Source: three-view drawing plus pictorial views. Frame: mm from the lowest corner of the part. Round coordinates to 2 decimals unless told otherwise and drop trailing zeros. Loops run counter-clockwise (first coordinate to the right, second up) from the corner with the lowest first, then second, coordinate; pieces in that order, holes last. Notation, with made-up numbers: (53, 18.25) -> (63, 18.25) arc R12 ccw to (63, 35.25) -> close; hole circle Ø8 at (-28, 29). An arc over 180 degrees is marked (long way). Put each result on its own line as item: value. Start each with the question number.
1. Material intervals for L1, parallel to Z at x = 0.85, y = 1.6; L2, parallel to Z at x = 5.7, y = 2.75; L3, parallel to Y at x = 2.85, z = 12.5, sorted ascending.
2. Cut plane A-A (z = 15). Return the cut outline in (x, y).
3. Contact query for a flat-ended pin moving along its axis: pin 1 (2 mm diameter, centred on y = 1.5, z = 19.5, fed in from +X). Output: stop coordinate, or through.
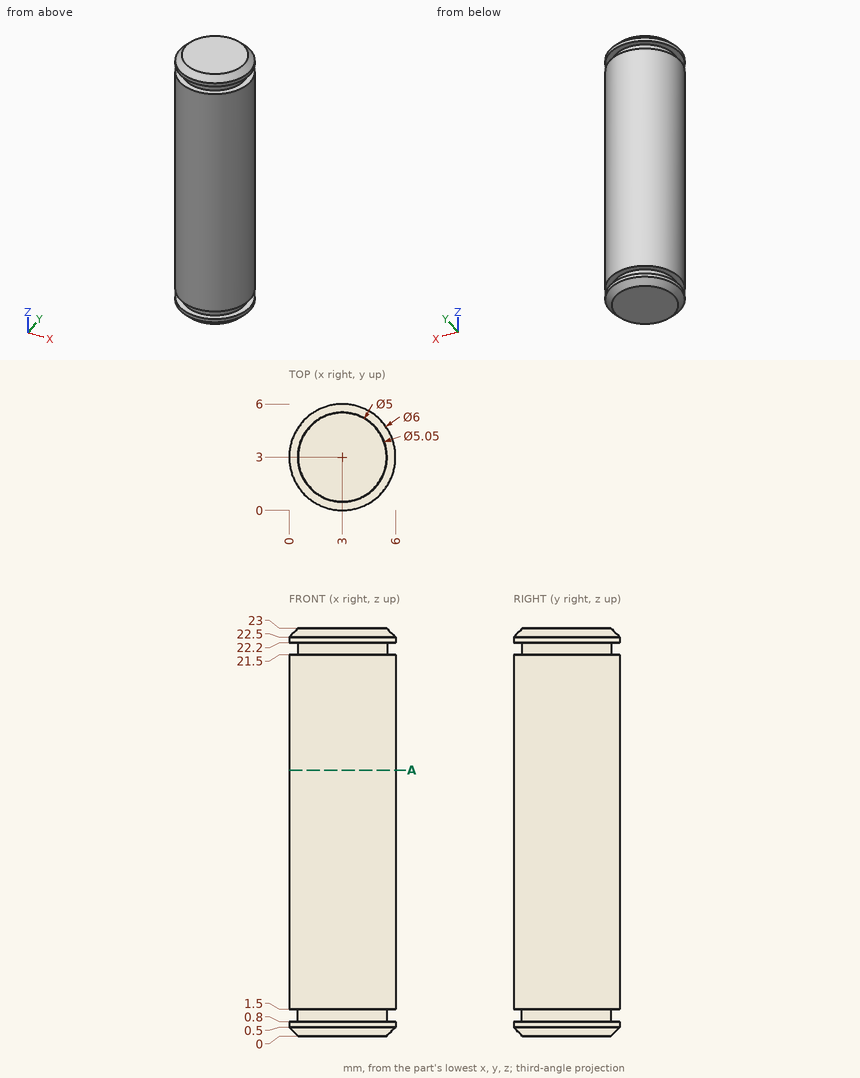
Solution:
1. L1: z = 0.07 to 0.8, 1.5 to 21.5, 22.2 to 22.93
1. L2: z = 0.21 to 0.8, 1.5 to 21.5, 22.2 to 22.79
1. L3: y = 0 to 6
2. outline: circle Ø6 at (3, 3)
3. pin 1: stops at x = 5.96
